Check sheet for the modelled part. Datum: model origin and axes. Units: mm. Face numbers are marked on the shaded views. A direction names the side the tool comes from. Round coordinates to 2 decimals unless told otherwise and drop trailing zeros. Write each loop counter-clockwise with the first axis right and the second up, starting at its lowest first coordinate (ties: lowest second). Pieces come first, ordered by that corner, then holes. Notation, with made-up numbers: (8.25, -25.75) - (18.25, -25.75) arc R27 ccw to (18.25, 13.25) - close; hole circle Ø1 at (31.25, -27). An arc over 180 degrees is marked (long way). Use one line per item in the form item = value. Start each with the question number.
1) Set-up check for the marked faces 5, 6 and 7: record each of +Z, -Z, +X, -X, +Y, -Y from which the full face is reachable in a straight line by a thin tool's end or side.
2) Section check A-A (y = 19). Record the boundary of the cut face in (x, z), then the cut area to 3 significant figures.
3) Section check D-D (x = 7.5). Record the boundary of the cut face in (y, z).
4) Section check B-B (x = -6.5). Record the boundary of the cut face in (y, z), then the cut area to 3 significant figures.
5) Draft check along Y on the marked faces 1, 2, 3 and 4. Enter one of: +Y half, -Y half, draft (parallel to the pull), parting line (faces both ways), or undercut.
6) Scan lines: probe 1 along Y at (x, z) = (20, 1.1); probe 2 along Y at (x, z) = (14, 1.05); probe 3 along Y at (x, z) = (7.5, 4.55). Record each from-to range of solid material in increasing order.
7) Section check C-C (x = 20). Record the boundary of the cut face in (y, z), then the cut area to 3 significant figures.
8) Gauge pin test, flat ends, axial feed: P1, Ø0.6, axis at x = 13, z = 4.5, coming from the -Y side; P2, Ø0.6, axis at x = -13, z = 4.5, coming from the +Y side; P3, Ø3, axis at x = 20, y = 13, coming from the +Z side. Record the tip position at first contact, or that the pin passes through.
from build123d import *

# Parameters (mm, degrees)
SKETCH1_W           = 44.8
SKETCH1_H           = 19.8
BOSS_EXTRUDE1_DEPTH = 5
SKETCH2_R           = 1.1
CUT_EXTRUDE1_DEPTH  = 13
SKETCH3_R           = 1.5
CUT_EXTRUDE2_DEPTH  = 10
SKETCH4_W           = 21
SKETCH4_H           = 12
CUT_EXTRUDE3_DEPTH  = 10
FILLET1_START       = 9.18
FILLET1_DEPTH       = 19.8
BOSS_EXTRUDE2_START = -5
SKETCH5_R           = 3.5
SKETCH5_R_2         = 1.5
BOSS_EXTRUDE2_DEPTH = 5


with BuildPart() as part:
    # Sketch1 → Boss-Extrude1 (new body)
    with BuildSketch(Plane.XY):
        with Locations((0, 19.08)):
            Rectangle(SKETCH1_W, SKETCH1_H)
    extrude(amount=BOSS_EXTRUDE1_DEPTH)

    # Sketch2 → Cut-Extrude1 (cut)
    with BuildSketch(Plane.XY.offset(5)):
        with Locations((-20, 25)):
            Circle(SKETCH2_R)
        with Locations((-20, 13)):
            Circle(SKETCH2_R)
        with Locations((20, 25)):
            Circle(SKETCH2_R)
        with Locations((20, 13)):
            Circle(SKETCH2_R)
    extrude(amount=-CUT_EXTRUDE1_DEPTH, mode=Mode.SUBTRACT)

    # Sketch3 → Cut-Extrude2 (cut)
    with BuildSketch(Plane.XY.offset(5)):
        with Locations((-14, 19)):
            Circle(SKETCH3_R)
        with Locations((14, 19)):
            Circle(SKETCH3_R)
    extrude(amount=-CUT_EXTRUDE2_DEPTH, mode=Mode.SUBTRACT)

    # Sketch4 → Cut-Extrude3 (cut)
    with BuildSketch(Plane.XY.offset(5)):
        with Locations((0, 19)):
            Rectangle(SKETCH4_W, SKETCH4_H)
    extrude(amount=-CUT_EXTRUDE3_DEPTH, mode=Mode.SUBTRACT)

    # Fillet1: read off the stored shape, not the designer's step
    # Fillet1 outline → Fillet1 (cut)
    with BuildSketch(Plane(origin=(0, 0, 0), x_dir=(1, 0, 0), z_dir=(0, 1, 0)).offset(FILLET1_START)):
        with BuildLine():
            Line((22.4, -5), (22.4, 0))
            ThreePointArc((22.4, 0), (14.477130086, -3.722813233), (5.816876048, -5))
            Line((5.816876048, -5), (22.4, -5))
        make_face()
        with BuildLine():
            Line((-22.4, -5), (-5.816876048, -5))
            ThreePointArc((-5.816876048, -5), (-14.477130086, -3.722813233), (-22.4, 0))
            Line((-22.4, 0), (-22.4, -5))
        make_face()
    extrude(amount=FILLET1_DEPTH, mode=Mode.SUBTRACT)

    # Sketch5 → Boss-Extrude2 (add)
    # profile 1 of 6: a face of its own
    with BuildSketch(Plane(origin=(0, 0, 0), x_dir=(-1, 0, 0), z_dir=(0, 0, -1)).offset(BOSS_EXTRUDE2_START)):
        with Locations((-14, 19)):
            Circle(SKETCH5_R)
        with Locations((-14, 19)):
            Circle(SKETCH5_R_2, mode=Mode.SUBTRACT)
    # profile 2 of 6: a face of its own
    with BuildSketch(Plane(origin=(0, 0, 0), x_dir=(-1, 0, 0), z_dir=(0, 0, -1)).offset(BOSS_EXTRUDE2_START)):
        with BuildLine():
            Line((-10.5, 22.5), (-14, 22.5))
            ThreePointArc((-14, 22.5), (-11.525126266, 21.474873734), (-10.5, 19))
            Line((-10.5, 19), (-10.5, 22.5))
        make_face()
    # profile 3 of 6: a face of its own
    with BuildSketch(Plane(origin=(0, 0, 0), x_dir=(-1, 0, 0), z_dir=(0, 0, -1)).offset(BOSS_EXTRUDE2_START)):
        with BuildLine():
            Line((-10.5, 15.5), (-10.5, 19))
            ThreePointArc((-10.5, 19), (-11.525126266, 16.525126266), (-14, 15.5))
            Line((-14, 15.5), (-10.5, 15.5))
        make_face()
    # profile 4 of 6: a face of its own
    with BuildSketch(Plane(origin=(0, 0, 0), x_dir=(-1, 0, 0), z_dir=(0, 0, -1)).offset(BOSS_EXTRUDE2_START)):
        with Locations((14, 19)):
            Circle(SKETCH5_R)
        with Locations((14, 19)):
            Circle(SKETCH5_R_2, mode=Mode.SUBTRACT)
    # profile 5 of 6: a face of its own
    with BuildSketch(Plane(origin=(0, 0, 0), x_dir=(-1, 0, 0), z_dir=(0, 0, -1)).offset(BOSS_EXTRUDE2_START)):
        with BuildLine():
            ThreePointArc((14, 15.5), (11.525126266, 16.525126266), (10.5, 19))
            Line((10.5, 19), (10.5, 15.5))
            Line((10.5, 15.5), (14, 15.5))
        make_face()
    # profile 6 of 6: a face of its own
    with BuildSketch(Plane(origin=(0, 0, 0), x_dir=(-1, 0, 0), z_dir=(0, 0, -1)).offset(BOSS_EXTRUDE2_START)):
        with BuildLine():
            ThreePointArc((10.5, 19), (11.525126266, 21.474873734), (14, 22.5))
            Line((14, 22.5), (10.5, 22.5))
            Line((10.5, 22.5), (10.5, 19))
        make_face()
    extrude(amount=BOSS_EXTRUDE2_DEPTH)


solid = part.part
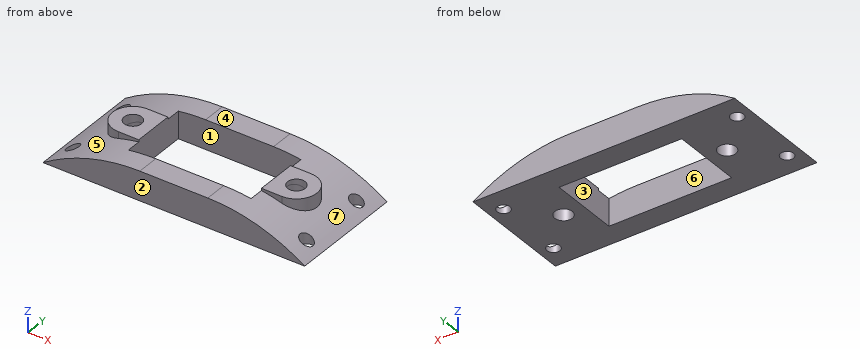
Results are:
q1.face_5 = +Z, -X
q1.face_6 = +Z, -Z
q1.face_7 = +Z, +X
q2.outline = (-22.4, 0) - (-15.5, 0) - (-15.5, 5) - (-17.5, 5) - (-17.5, 2.63) arc R30 ccw to start; (-12.5, 0) - (-10.5, 0) - (-10.5, 5) - (-12.5, 5) - close; (10.5, 0) - (12.5, 0) - (12.5, 5) - (10.5, 5) - close; (15.5, 0) - (22.4, 0) arc R30 ccw to (17.5, 2.63) - (17.5, 5) - (15.5, 5) - close
q2.area = 53.9 mm²
q3.outline = (9.18, 0) - (13, 0) - (13, 4.95) - (9.18, 4.95) - close; (25, 0) - (28.98, 0) - (28.98, 4.95) - (25, 4.95) - close
q4.outline = (9.18, 0) - (13, 0) - (13, 4.99) - (9.18, 4.99) - close; (25, 0) - (28.98, 0) - (28.98, 4.99) - (25, 4.99) - close
q4.area = 38.9 mm²
q5.face_1 = undercut
q5.face_2 = -Y half
q5.face_3 = undercut
q5.face_4 = draft
q6.probe_1 = 9.18 to 11.9, 14.1 to 23.9, 26.1 to 28.98
q6.probe_2 = 9.18 to 17.5, 20.5 to 28.98
q6.probe_3 = 9.18 to 13, 25 to 28.98
q7.outline = (9.18, 0) - (11.9, 0) - (11.9, 1.44) - (9.18, 1.44) - close; (14.1, 0) - (23.9, 0) - (23.9, 1.44) - (14.1, 1.44) - close; (26.1, 0) - (28.98, 0) - (28.98, 1.44) - (26.1, 1.44) - close
q7.area = 22.1 mm²
q8.P1 = 15.5
q8.P2 = 22.5
q8.P3 = 2.19
